from build123d import *

# Parameters (mm, degrees)
SKETCH1_R               = 2.75
BOSS_EXTRUDE1_DEPTH     = 19.2
SKETCH13_OUTSIDE_W      = 41
SKETCH13_OUTSIDE_H      = 115.36
CUT_EXTRUDE4_DEPTH      = 84.275329734
CUT_EXTRUDE4_DEPTH_BACK = 84.275329734
CUT_EXTRUDE2_DEPTH      = 4
SKETCH4_R               = 4.05
CUT_EXTRUDE3_DEPTH      = 20
FILLET4_R               = 10
BOSS_EXTRUDE2_REACH     = 83.7
SKETCH9_R               = 13
SKETCH10_R              = 8
BOSS_EXTRUDE3_DEPTH     = 27
DRAFT1_ANGLE            = -3
FILLET5_R               = 25
SKETCH14_R              = 2
CUT_EXTRUDE5_DEPTH      = 4
FILLET6_R               = 1.5


with BuildPart() as part:
    # Sketch1 → Boss-Extrude1 (new body)
    with BuildSketch(Plane.XY):
        with BuildLine():
            Line((-7.5, 70.183778092), (-10, 11.180339887))
            ThreePointArc((-10, 11.180339887), (0, -15), (10, 11.180339887))
            Line((10, 11.180339887), (7.5, 70.183778092))
            ThreePointArc((7.5, 70.183778092), (0, 77.372729176), (-7.5, 70.183778092))
        make_face()
        with Locations((0, 69.866)):
            Circle(SKETCH1_R, mode=Mode.SUBTRACT)
    extrude(amount=BOSS_EXTRUDE1_DEPTH)

    # Sketch13 outside → Cut-Extrude4 (cut, two sides)
    with BuildSketch(Plane(origin=(10.454946348, 0.442980387, 0), x_dir=(0, 0, -1), z_dir=(0.9991035808766652, 0.042332430587259585, 0))) as cut_extrude4_sk:
        with Locations((-9.6, 31.158)):
            Rectangle(SKETCH13_OUTSIDE_W, SKETCH13_OUTSIDE_H)
        Polygon((-16.15, 77.310099957), (-16.15, 57.310099957), (-3.05, 57.310099957), (-3.05, 77.310099957), (0, 77.310099957), (0, 52.310099957), (-4.6, 39.671703828), (-4.6, -15), (-14.6, -15), (-14.6, 39.671703828), (-19.2, 52.310099957), (-19.2, 77.310099957), align=None, mode=Mode.SUBTRACT)
    extrude(amount=CUT_EXTRUDE4_DEPTH, mode=Mode.SUBTRACT)
    extrude(cut_extrude4_sk.sketch, amount=-CUT_EXTRUDE4_DEPTH_BACK, mode=Mode.SUBTRACT)

    # Sketch3 → Cut-Extrude2 (cut)
    with BuildSketch(Plane.XY.offset(14.6)):
        Polygon((0, 7.332348419), (-6.35, 3.666174209), (-6.35, -3.666174209), (0, -7.332348419), (6.35, -3.666174209), (6.35, 3.666174209), align=None)
    extrude(amount=-CUT_EXTRUDE2_DEPTH, mode=Mode.SUBTRACT)

    # Sketch4 → Cut-Extrude3 (cut)
    with BuildSketch(Plane.XY.offset(10.6)):
        Circle(SKETCH4_R)
    extrude(amount=-CUT_EXTRUDE3_DEPTH, mode=Mode.SUBTRACT)

    # Fillet4
    fillet4_edges = [part.edges().sort_by_distance(p)[0] for p in [
        (10, 11.180339887, 9.6),
        (-10, 11.180339887, 9.6),
    ]]
    fillet(fillet4_edges, radius=FILLET4_R)

    # Boss-Extrude2: up to this plane
    boss_extrude2_end = Plane(origin=(-17.286936373, 38.974843589, 4.6), z_dir=(0, 0, -1))
    # Sketch9 → Boss-Extrude2 (add, up to the surface)
    with BuildSketch(Plane(origin=(0, 2.715435503, -10.4), x_dir=(-1, 0, 0), z_dir=(0, 0.17364817766692367, -0.9848077530122092)), mode=Mode.PRIVATE) as boss_extrude2_sk1:
        with Locations(Location((0, -0.868240888, 0), (0, 0, 90))):
            Circle(SKETCH9_R)
    boss_extrude2_tool1 = split(extrude(boss_extrude2_sk1.sketch, amount=-BOSS_EXTRUDE2_REACH, mode=Mode.PRIVATE), bisect_by=boss_extrude2_end, keep=Keep.BOTH, mode=Mode.PRIVATE)
    add(boss_extrude2_tool1.solids().sort_by_distance((0, 1.860385, -10.550768))[0])

    # Sketch10 → Boss-Extrude3 (add)
    with BuildSketch(Plane(origin=(0, 1.860385145, -10.550768448), x_dir=(-1, 0, 0), z_dir=(0, 0.17364817766692367, -0.9848077530122092))):
        with Locations(Location((0, 0, 0), (0, 0, 90))):
            Circle(SKETCH10_R)
    extrude(amount=BOSS_EXTRUDE3_DEPTH)

    # Draft1
    draft1_faces = [part.faces().sort_by_distance(p)[0] for p in [
        (0, -12.485127219, -4.05734127),
    ]]
    draft(draft1_faces, Plane(origin=(0, 1.860385145, -10.550768448), x_dir=(0, -0.9848077530122092, -0.17364817766692367), z_dir=(0, 0.17364817766692367, -0.9848077530122092)), DRAFT1_ANGLE)

    # Fillet5
    fillet5_edges = [part.edges().sort_by_distance(p)[0] for p in [
        (-0.01578265, 39.706629492, 4.6),
        (-0.01578265, 39.706629492, 14.6),
        (-0.014820438, 52.356405855, 19.2),
        (-0.014820438, 52.356405855, 0),
    ]]
    fillet(fillet5_edges, radius=FILLET5_R)

    # Sketch14 → Cut-Extrude5 (cut)
    with BuildSketch(Plane(origin=(0, 6.548885942, -37.140577779), x_dir=(-1, 0, 0), z_dir=(0, 0.17364817766692367, -0.9848077530122092))):
        with Locations(Location((-3.464101615, 2, 0), (0, 0, 90))):
            Circle(SKETCH14_R)
        with Locations(Location((3.464101615, 2, 0), (0, 0, 90))):
            Circle(SKETCH14_R)
        with Locations(Location((0, -4, 0), (0, 0, 90))):
            Circle(SKETCH14_R)
    extrude(amount=-CUT_EXTRUDE5_DEPTH, mode=Mode.SUBTRACT)

    # Fillet6
    fillet6_edges = [part.edges().sort_by_distance(p)[0] for p in [
        (-9.82e-07, -13.079573194, 4.6),
        (-0.014439768, 57.360908102, 3.05),
        (-0.014439768, 57.360908102, 16.15),
    ]]
    fillet(fillet6_edges, radius=FILLET6_R)


solid = part.part
Design review of the part built by this model. Coordinates are the model's own, in mm. A direction names the side the tool comes from. Round coordinates to 2 decimals unless told otherwise and drop trailing zeros. Loops run counter-clockwise (first coordinate to the right, second up) from the corner with the lowest first, then second, coordinate; pieces in that order, holes last. Notation, with made-up numbers: (-37.75, 24.25) - (-27.75, 24.25) arc R17 cw to (-27.75, 28.25) - close; hole circle Ø5 at (78, 51.5). An arc over 180 degrees is marked (long way). One line per question, with ' | ' between items.
1. We need section B-B, the plane y = 31. State the section outline as (x, z) points, and give its area (3 significant figures).
Results are:
outline: (-9.16, 4.6) - (9.16, 4.6) - (9.16, 14.6) - (-9.16, 14.6) - close | area: 183 mm²
2. We need section A-A, the plane z = 12. State the section outline as (x, y) points.
Results are:
outline: (-11.9, 9.13) arc R15 ccw (long way) to (11.9, 9.13) arc R10 cw to (9.85, 14.79) - (8.03, 57.7) - (-8.06, 57.02) - (-9.85, 14.79) arc R10 cw to start; hole (-6.35, -3.67) - (0, -7.33) - (6.35, -3.67) - (6.35, 3.67) - (0, 7.33) - (-6.35, 3.67) - close
3. For faces 4 (the face through (-0.31, 52.35, 0.39)), 5 (the face through (0, 65, 0)), 6 (the face through (-0.145, 57.783, 3.501)), 7 (the face through (5.96, 7.37, -9.58)), 8 (the face through (-3.131, 5.525, 12.628)), list the 3-axis set-ups (+Z, -Z, +X, -X, +Y, -Y) from which the entire face can be reached by the end or side of a thin tool; tool diameter is ignored.
Results are:
face 4: -Z, +X | face 5: -Z, +X, -X, +Y | face 6: -X, +Y | face 7: none | face 8: +Z
4. For L1, parallel to Z at x = -7.5, y = 66; L2, parallel to X at y = 6.5, z = 11, list the stretches that pass through material, from the lowest coordinate up. Write a range as [from, to].
Results are:
L1: z = [0, 3.05], [16.15, 19.2] | L2: x = [-13.52, -1.44], [1.44, 13.52]
5. Draft analysis for pull direction X (two halves, no side actions). For faces 1 (the face through (-7.81, 2.46, -23.96)), 2 (the face through (3.49, 7.8, -32.86)), 3 (the face through (0, 66, 16.15)), state which applies: released by +X, released by -X, zero draft, split by the parting line, or undercut.
Results are:
face 1: split by the parting line | face 2: undercut | face 3: zero draft
6. Clearance check with flat-ended pins moving along their axes: P1, Ø6, axis at x = -9, y = 31, coming from the +Z side; P2, Ø15, axis at x = -5, y = 22.5, coming from the -Z side; P3, Ø1.2, axis at y = -1, z = 12, coming from the +X side; P4, Ø3.5, axis at x = 0, y = 69.866, coming from the +Z side. State where each tip first meets the part, or that it passes through.
Results are:
P1: stops at z = 14.6 | P2: stops at z = 4.6 | P3: stops at x = 14.99 | P4: passes through
